Read the model definition and answer for the solid it produces. Units are mm, in the model's axes. A direction names the side the tool comes from. Give positions to 0.01 mm unless a question says otherwise; leave off trailing zeros. Write each loop counter-clockwise with the first axis right and the second up, starting at its lowest first coordinate (ties: lowest second). Pieces come first, ordered by that corner, then holes. Notation, with made-up numbers: M 88.25,-22 L 99.25,-22 A37 ccw 99.25,15 Z; hole C 32.25,84.5 d7. An arc over 180 degrees is marked long. Put each result on its own line as item: value.
from build123d import *

# Parameters (mm, degrees)
BOSS_EXTRUDE1_DEPTH                                 = 5
CSK_FOR_M3_COUNTERSUNK_FLAT_HEAD_SCREW1_D           = 3.4
CSK_FOR_M3_COUNTERSUNK_FLAT_HEAD_SCREW1_CSINK_D     = 6.3
CSK_FOR_M3_COUNTERSUNK_FLAT_HEAD_SCREW1_CSINK_ANGLE = 90
BOSS_EXTRUDE2_DEPTH                                 = 5
FILLET1_R                                           = 2
SKETCH8_R                                           = 8
CUT_EXTRUDE1_DEPTH                                  = 56
RIB1_REACH                                          = 78.426
SKETCH10_WALL_W                                     = 176.100560442
SKETCH10_WALL_H                                     = 4
SKETCH11_W                                          = 4
SKETCH11_H                                          = 4
CUT_EXTRUDE2_DEPTH                                  = 8
CIRPATTERN1_COUNT                                   = 4


with BuildPart() as part:
    # Sketch2 → Boss-Extrude1 (new body)
    with BuildSketch(Plane(origin=(0, 0, 0), x_dir=(1, 0, 0), z_dir=(0, 1, 0))):
        with BuildLine():
            Line((-20, 30), (20, 30))
            Line((20, 30), (45, 18.342308546))
            Line((45, 18.342308546), (45, 6))
            Line((45, 6), (29, 6))
            ThreePointArc((29, 6), (23, 0), (29, -6))
            Line((29, -6), (45, -6))
            Line((45, -6), (45, -18.342308546))
            Line((45, -18.342308546), (20, -30))
            Line((20, -30), (-20, -30))
            Line((-20, -30), (-45, -18.342308546))
            Line((-45, -18.342308546), (-45, -6))
            Line((-45, -6), (-29, -6))
            ThreePointArc((-29, -6), (-23, 0), (-29, 6))
            Line((-29, 6), (-45, 6))
            Line((-45, 6), (-45, 18.342308546))
            Line((-45, 18.342308546), (-20, 30))
        make_face()
    extrude(amount=BOSS_EXTRUDE1_DEPTH)

    # CSK for M3 Countersunk Flat Head Screw1 (through all)
    with Locations(Plane(origin=(0, 5, 0), x_dir=(1, 0, 0), z_dir=(0, 1, 0))):
        with Locations((-30, 15), (30, -15), (30, 15), (-30, -15)):
            CounterSinkHole(CSK_FOR_M3_COUNTERSUNK_FLAT_HEAD_SCREW1_D / 2, CSK_FOR_M3_COUNTERSUNK_FLAT_HEAD_SCREW1_CSINK_D / 2, counter_sink_angle=CSK_FOR_M3_COUNTERSUNK_FLAT_HEAD_SCREW1_CSINK_ANGLE)

    # Sketch6 → Boss-Extrude2 (add)
    with BuildSketch(Plane(origin=(0, 5, 0), x_dir=(1, 0, 0), z_dir=(0, 1, 0))):
        with BuildLine():
            Line((-8, -20), (8, -20))
            ThreePointArc((8, -20), (16.485281374, -16.485281374), (20, -8))
            Line((20, -8), (20, 8))
            ThreePointArc((20, 8), (16.485281374, 16.485281374), (8, 20))
            Line((8, 20), (-8, 20))
            ThreePointArc((-8, 20), (-16.485281374, 16.485281374), (-20, 8))
            Line((-20, 8), (-20, -8))
            ThreePointArc((-20, -8), (-16.485281374, -16.485281374), (-8, -20))
        make_face()
    extrude(amount=BOSS_EXTRUDE2_DEPTH)

    # Fillet1
    fillet1_edges = [part.edges().sort_by_distance(p)[0] for p in [
        (-16.485281374, 5, 16.485281374),
        (0, 5, 20),
        (16.485281374, 5, 16.485281374),
        (20, 5, 0),
        (16.485281374, 5, -16.485281374),
        (0, 5, -20),
        (-16.485281374, 5, -16.485281374),
        (-20, 5, 0),
    ]]
    fillet(fillet1_edges, radius=FILLET1_R)

    # Sketch8 → Cut-Extrude1 (cut, through all)
    with BuildSketch(Plane.XZ):
        with Locations(Location((0, 0, 0), (0, 0, 270))):
            Circle(SKETCH8_R)
    extrude(amount=-CUT_EXTRUDE1_DEPTH, mode=Mode.SUBTRACT)

    # Sketch9 → Revolve1 (revolve)
    with BuildSketch(Plane.XY, mode=Mode.PRIVATE) as revolve1_sk:
        with BuildLine():
            Line((-8, 10), (-17.5, 10))
            Line((-17.5, 10), (-17.5, 20))
            Line((-17.5, 20), (-20, 27))
            Line((-20, 27), (-20, 40))
            Line((-20, 40), (-13.1, 40))
            ThreePointArc((-13.1, 40), (-12.1, 41), (-13.1, 42))
            Line((-13.1, 42), (-15, 42))
            Line((-15, 42), (-15, 54))
            Line((-15, 54), (-10, 54))
            Line((-10, 54), (-10, 46))
            Line((-10, 46), (-6, 46))
            Line((-6, 46), (-6, 34))
            Line((-6, 34), (-8, 28))
            Line((-8, 28), (-8, 10))
        make_face()
    revolve(revolve1_sk.sketch.rotate(Axis((0, -7.60274032, 0), (0, 1, 0)), 270), axis=Axis((0, -7.60274032, 0), (0, 1, 0)))

    # Sketch10 wall → Rib1 (add, up to next)
    with BuildSketch(Plane(origin=(0, 14.628473456, 23.510169091), x_dir=(0, 0.906307787042, -0.42261826173), z_dir=(0, 0.42261826173, 0.906307787042)), mode=Mode.PRIVATE) as rib1_sk1:
        Rectangle(SKETCH10_WALL_W, SKETCH10_WALL_H)
    rib1_tool1 = extrude(rib1_sk1.sketch, amount=-RIB1_REACH, mode=Mode.PRIVATE) - part.part
    rib1 = rib1_tool1.solids().sort_by_distance((0, 14.628473456, 23.510169091))[0]
    add(rib1)

    # Mirror1: Rib1 across plane
    add(rib1.mirror(Plane.XY))

    # Sketch11 → Cut-Extrude2 (cut)
    with BuildSketch(Plane(origin=(0, 40, 0), x_dir=(1, 0, 0), z_dir=(0, 1, 0))):
        with Locations((18, 0)):
            Rectangle(SKETCH11_W, SKETCH11_H)
    cut_extrude2 = extrude(amount=-CUT_EXTRUDE2_DEPTH, mode=Mode.SUBTRACT)

    # CirPattern1: Cut-Extrude2 ×4 about axis
    cirpattern1_axis = Axis((0, 0, 0), (0, 1, 0))
    for i in range(1, CIRPATTERN1_COUNT):
        add(cut_extrude2.rotate(cirpattern1_axis, i * 360 / CIRPATTERN1_COUNT), mode=Mode.SUBTRACT)


solid = part.part
(1) Given pin 1 Ø1.5 at (y, z) = (9, -3.5) entering from -X; pin 2 Ø2 at (y, z) = (34, 0.5) entering from -X; pin 3 Ø2.5 at (x, y) = (-35, 2) entering from +Z, each flat-ended and moving along its own axis, determine where each tip first touches the part or whether it passes through.
Result:
pin 1: stops at x = -20
pin 2: stops at x = -16
pin 3: stops at z = 23.59
(2) Section A-A on x = 34.5 is taken. Determine the outline of the cut face in (y, z).
Result:
outline: M 0,-23.24 L 5,-23.24 L 5,-6 L 0,-6 Z; M 0,6 L 5,6 L 5,23.24 L 0,23.24 Z
(3) Section C-C on y = 50.5 is taken. Determine the outline of the cut face in (x, z), and give its area (3 significant figures).
Result:
outline: C 0,0 d30; hole C 0,0 d20
area: 393 mm²
(4) Straight lines are drawn through the part: line 1 along X through (y, z) = (1, 15); line 2 along X through (y, z) = (7.25, 0); line 3 along X through (y, z) = (47.75, 0). For each, find the intervals that lie inside material, in ascending order. Write a range as from..to.
Result:
line 1: x = -45..-31.7, -28.3..28.3, 31.7..45
line 2: x = -20..-8, 8..20
line 3: x = -15..-10, 10..15
(5) For a pull along X with two mould halves and no side action, classify faces 6 (the face through (18, 36, -2)), 7 (the face through (-45, 2, -12)), 8 (the face through (9.76, 49.94, 2.17)) as +X half, -X half, draft (parallel to the pull), parting line (faces both ways), or undercut.
Result:
face 6: draft
face 7: -X half
face 8: undercut
(6) Which of the six approach directions +Z, -Z, +X, -X, +Y, -Y give full straight-line access (tool end or side, diameter ignored) to faces 1 (the face through (-17.496, 15.07, -0.357)), 2 (the face through (-2, 36, 18)), 3 (the face through (4.96, 5.57, -20.6)), 4 (the face through (-20, 8, 0)), 5 (the face through (-5.04, 5.57, -20.6))?
Result:
face 1: -X
face 2: +Z, +Y
face 3: -Z, +X, +Y
face 4: +Z, -Z, -X, +Y
face 5: -Z, -X, +Y
(7) Section B-B on x = -30 is taken. Determine the outline of the cut face in (y, z), and give its area (3 significant figures).
Result:
outline: M 0,-25.34 L 5,-25.34 L 5,-18.15 L 3.55,-16.7 L 0,-16.7 Z; M 0,-13.3 L 3.55,-13.3 L 5,-11.85 L 5,-6 L 0,-6 Z; M 0,6 L 5,6 L 5,11.85 L 3.55,13.3 L 0,13.3 Z; M 0,16.7 L 3.55,16.7 L 5,18.15 L 5,25.34 L 0,25.34 Z
area: 155 mm²
(8) Section D-D on z = 25.5 is taken. Determine the outline of the cut face in (x, y), and give its area (3 significant figures).
Result:
outline: M -29.65,0 L 29.65,0 L 29.65,5 L 2,5 L 2,10.36 L -2,10.36 L -2,5 L -29.65,5 Z
area: 318 mm²
